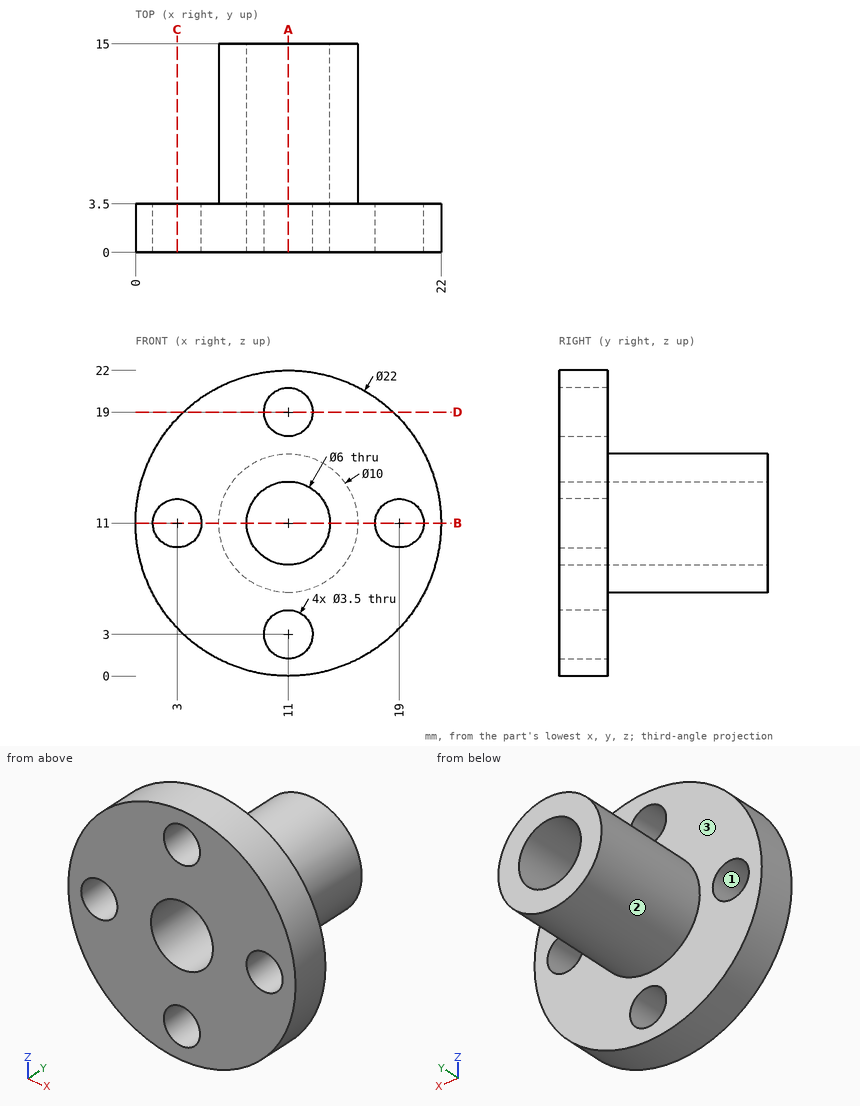
Here's the drawing with two shaded views (mm, measured from the low corner). I have some questions. Coordinates: 2 decimals unless noted, no trailing zeros. Order: outer loops, then holes, each group sorted by start corner. A loop starts at its lowest first (then second) coordinate and runs counter-clockwise, first axis right, second up. Notation, with made-up numbers: M -21,-15 L 37,-15 A22 ccw 37,5 Z; hole C 84.25,44 d2. An arc over 180 degrees is marked long. Write item = value, one per line.
(1) Suppose I cut it at D-D on z = 19. Please give me the cut outline in (x, y), plus the area to 3 significant figures.
Results are:
outline = M 3.45,0 L 9.25,0 L 9.25,3.5 L 3.45,3.5 Z; M 12.75,0 L 18.55,0 L 18.55,3.5 L 12.75,3.5 Z
area = 40.6 mm2
(2) If we mould it in two halves opening along Z, with no side actions, what happens to the marked faces 1, 2 and 3? For each: pulls with the +Z half, pulls with the -Z half, needs draft (parallel to the pull), parting line crosses it, or undercut.
Results are:
face_1 = undercut
face_2 = parting line crosses it
face_3 = needs draft
(3) I need wall thicknesses on line 1 along X through (y, z) = (7, 11); line 2 along Y through (x, z) = (10, 17.25); line 3 along Z through (x, y) = (10.5, 4). Which ranges of each line are inside material? Lowest first, please. Write a range as [from, to].
Results are:
line_1 = [6, 8], [14, 16]
line_2 = [0, 3.5]
line_3 = [6.03, 8.04], [13.96, 15.97]
(4) Suppose I cut it at C-C on x = 3. Please give me the cut outline in (y, z).
Results are:
outline = M 0,3.45 L 3.5,3.45 L 3.5,9.25 L 0,9.25 Z; M 0,12.75 L 3.5,12.75 L 3.5,18.55 L 0,18.55 Z
(5) For pin 1 Ø5.5 at (x, z) = (19, 11) entering from +Y; pin 2 Ø3 at (x, z) = (11, 3) entering from -Y; pin 3 Ø1.5 at (x, y) = (10, 7.5) entering from +Z; pin 4 Ø6 at (x, y) = (16.5, 8.5) entering from -Z, each with a flat end and sliding along its axis, tell me the tip position at first contact or that it passes through.
Results are:
pin_1 = 3.5
pin_2 = through
pin_3 = 15.99
pin_4 = 6.67
(6) Suppose I cut it at B-B on z = 11. Please give me the cut outline in (x, y), plus the area to 3 significant figures.
Results are:
outline = M 0,0 L 1.25,0 L 1.25,3.5 L 0,3.5 Z; M 4.75,0 L 8,0 L 8,15 L 6,15 L 6,3.5 L 4.75,3.5 Z; M 14,0 L 17.25,0 L 17.25,3.5 L 16,3.5 L 16,15 L 14,15 Z; M 20.75,0 L 22,0 L 22,3.5 L 20.75,3.5 Z
area = 77.5 mm2
(7) Suppose I cut it at A-A on x = 11. Please give me the cut outline in (y, z), plus the area to 3 significant figures.
Results are:
outline = M 0,0 L 3.5,0 L 3.5,1.25 L 0,1.25 Z; M 0,4.75 L 3.5,4.75 L 3.5,6 L 15,6 L 15,8 L 0,8 Z; M 0,14 L 15,14 L 15,16 L 3.5,16 L 3.5,17.25 L 0,17.25 Z; M 0,20.75 L 3.5,20.75 L 3.5,22 L 0,22 Z
area = 77.5 mm2
